Work out the finished part from the listing and answer in its coordinate system (mm). A direction names the side the tool comes from. Coordinates: 2 decimals unless noted, no trailing zeros. Order: outer loops, then holes, each group sorted by start corner. A loop starts at its lowest first (then second) coordinate and runs counter-clockwise, first axis right, second up. Notation, with made-up numbers: M -19,60.5 L 36,60.5 A23 cw 36,90.5 Z; hole C -6,-4 d4. An arc over 180 degrees is marked long. Answer in a Markdown table with one row per item. Add a question column.
Item 1: The mould has two halves that part along Y. Classify faces 1 (the face through (99, 41.6, 10)), 2 (the face through (127.05, 40.93, 8.65)), 3 (the face through (35, 62, 8)): released by +Y, released by -Y, zero draft, split by the parting line, or undercut.
Item 2: The part is cut by section A-A (z = 3.5). Write down the section's boundary in (x, y).
Item 3: Which of the six approach directions +Z, -Z, +X, -X, +Y, -Y give full straight-line access (tool end or side, diameter ignored) to faces 4 (the face through (1.972, 91.669, 8.526)), 5 (the face through (38, 64, 11)), 6 (the face through (125.1, 68.9, 10)), 7 (the face through (9, 102.5, 10))?
Item 4: Flat-ended cylindrical pins translate along their axes: pin 1 Ø3.5 at (y, z) = (99, 13) entering from -X; pin 2 Ø5 at (x, z) = (26, 2) entering from -Y; pin 3 Ø3.5 at (x, y) = (123.5, 98) entering from -Z. Find the tip coordinate at first contact, or state that the pin passes through.
Item 5: Consider line 1 (X direction, y = 87.5, z = 6); line 2 (Y direction, x = 123.4, z = 13.95); line 3 (Y direction, x = 123.4, z = 8). Determine where each line is inside the solid, lowest interval first. Write a range as from..to.
Item 6: The part is cut by section C-C (y = 55.5). Write down the section's boundary in (x, z), then the cut area to 3 significant figures.
Item 7: The part is cut by section D-D (y = 84). Write down the section's boundary in (x, z).
Item 8: The part is cut by section B-B (y = 70.6). Write down the section's boundary in (x, z), then the cut area to 3 significant figures.
from build123d import *

# Parameters (mm, degrees)
SKETCH_R        = 2.25
PAD_DEPTH       = 16
POCKET_DEPTH    = 21
SKETCH002_R     = 1.75
POCKET001_DEPTH = 23
SKETCH003_R     = 1.75
SKETCH003_R_2   = 2.15
POCKET002_DEPTH = 46
SKETCH005_R     = 8
POCKET004_DEPTH = 5
POCKET005_DEPTH = 4.4
SKETCH007_W     = 10.5
SKETCH007_H     = 21
POCKET006_DEPTH = 6
POCKET007_DEPTH = 18
SKETCH009_R     = 1.75
POCKET008_DEPTH = 86


with BuildPart() as part:
    # Sketch → Pad (new body)
    with BuildSketch(Plane.XY):
        with BuildLine():
            Line((126.5, 107.1), (-1.5, 107.1))
            Line((-1.5, 107.1), (-1.5, 104.4))
            Line((-1.5, 104.4), (-5.7, 104.4))
            Line((-5.7, 104.4), (-5.7, 102.4))
            Line((-5.7, 102.4), (0, 102.4))
            Line((0, 102.4), (0, 62))
            Line((0, 62), (70.6, 62))
            Line((70.6, 62), (70.6, 36))
            Line((70.6, 36), (75.6, 36))
            Line((75.6, 36), (133.571068, 36))
            ThreePointArc((133.571068, 36), (133.891989, 37.231735), (134, 38.5))
            Line((134, 38.5), (134, 99.6))
            ThreePointArc((134, 99.6), (131.803301, 104.903301), (126.5, 107.1))
        make_face()
        with Locations((123.4, 70.6)):
            Circle(SKETCH_R, mode=Mode.SUBTRACT)
    extrude(amount=PAD_DEPTH)

    # Sketch001 (on DatumPlane) → Pocket (cut)
    with BuildSketch(Plane.XY.offset(5)):
        Polygon((128.6, 101.8), (131, 101.8), (131, 79.9), (120.7, 79.9), (120.7, 93.6), (120.7, 93.9), (124.3, 93.9), (128.6, 93.9), align=None)
        with BuildLine():
            add(Edge.make_bspline(
                [(13.289069, 102.5), (27.487875, 102.5), (63.575842, 75.600151), (81.110251, 102.5), (98.331885, 102.5)],
                knots=[0, 0, 0, 0, 0.5, 1, 1, 1, 1], degree=3))
            Line((98.331885, 102.5), (109.7, 102.5))
            Line((109.7, 102.5), (109.7, 58))
            Line((109.7, 58), (122, 58))
            Line((122, 58), (122, 41.6))
            Line((122, 41.6), (80, 41.6))
            Line((80, 41.6), (75.6, 41.6))
            Line((75.6, 41.6), (75.6, 67))
            Line((75.6, 67), (4, 67))
            Line((4, 67), (4, 102.5))
            Line((4, 102.5), (13.289069, 102.5))
        make_face()
    extrude(amount=POCKET_DEPTH, mode=Mode.SUBTRACT)

    # Sketch002 → Pocket001 (cut)
    with BuildSketch(Plane.YZ):
        with Locations((12, 8)):
            Circle(SKETCH002_R)
        with Locations((60, 8)):
            Circle(SKETCH002_R)
        with Locations((90, 8)):
            Circle(SKETCH002_R)
    extrude(amount=POCKET001_DEPTH, mode=Mode.SUBTRACT)

    # Sketch003 → Pocket002 (cut)
    with BuildSketch(Plane.XZ):
        with Locations((58.6, 8)):
            Circle(SKETCH003_R)
        with Locations((8, 8)):
            Circle(SKETCH003_R)
        with Locations((125, 8)):
            Circle(SKETCH003_R_2)
    extrude(amount=-POCKET002_DEPTH, mode=Mode.SUBTRACT)

    # Sketch005 (on DatumPlane) → Pocket004 (cut, symmetric)
    with BuildSketch(Plane.XY.offset(5)):
        with Locations((123.4, 70.6)):
            Circle(SKETCH005_R)
    extrude(amount=POCKET004_DEPTH, both=True, mode=Mode.SUBTRACT)

    # Sketch006 (on DatumPlane) → Pocket005 (cut)
    with BuildSketch(Plane.XY.offset(16)):
        Polygon((116.7, 102.3), (124.3, 102.3), (124.3, 93.9), (124.3, 93.6), (120.7, 93.6), (116.7, 93.6), align=None)
    extrude(amount=-POCKET005_DEPTH, mode=Mode.SUBTRACT)

    # Sketch007 (on DatumPlane) → Pocket006 (cut)
    with BuildSketch(Plane.XY.offset(5)):
        with Locations((125.75, 91.3)):
            Rectangle(SKETCH007_W, SKETCH007_H)
    extrude(amount=-POCKET006_DEPTH, mode=Mode.SUBTRACT)

    # Sketch008 (on DatumPlane) → Pocket007 (cut)
    with BuildSketch(Plane.XY.offset(5)):
        Polygon((127.328613, 102.8), (132, 102.8), (132, 79.494476), (119.5, 79.494476), (119.5, 94.960373), (127.328613, 94.960373), align=None)
    extrude(amount=POCKET007_DEPTH, mode=Mode.SUBTRACT)

    # Sketch009 → Pocket008 (cut)
    with BuildSketch(Plane.XZ):
        with Locations((58.6, 8)):
            Circle(SKETCH009_R)
        with BuildLine():
            ThreePointArc((33, 16), (38, 11), (43, 16))
            Line((43, 16), (43, 31.673506))
            ThreePointArc((43, 31.673506), (38, 36.673506), (33, 31.673506))
            Line((33, 31.673506), (33, 16))
        make_face()
    extrude(amount=-POCKET008_DEPTH, mode=Mode.SUBTRACT)


solid = part.part
Reply:
| question | item | result |
|---|---|---|
| 1 | face 1 | undercut |
| 1 | face 2 | zero draft |
| 1 | face 3 | released by -Y |
| 2 | outline | M -5.7,102.4 L 0,102.4 L 0,62 L 70.6,62 L 70.6,36 L 133.57,36 A7.5 ccw 134,38.5 L 134,99.6 A7.5 ccw 126.5,107.1 L -1.5,107.1 L -1.5,104.4 L -5.7,104.4 Z; hole C 123.4,70.6 d16; hole M 120.5,80.8 L 131,80.8 L 131,101.8 L 120.5,101.8 Z |
| 3 | face 4 | -X |
| 3 | face 5 | +Z, -Y |
| 3 | face 6 | -Z |
| 3 | face 7 | +Z |
| 4 | pin 1 | stops at x = 0 |
| 4 | pin 2 | stops at y = 62 |
| 4 | pin 3 | stops at z = 5 |
| 5 | line 1 | x = 0..4, 109.7..119.5, 132..134 |
| 5 | line 2 | y = 36..68.35, 72.85..79.49, 102.3..107.1 |
| 5 | line 3 | y = 46..62.6, 78.6..79.49, 94.96..107.1 |
| 6 | outline | M 70.6,0 L 134,0 L 134,16 L 122,16 L 122,5 L 75.6,5 L 75.6,16 L 70.6,16 Z |
| 6 | area | 504 mm2 |
| 7 | outline | M 0,0 L 120.5,0 L 120.5,5 L 119.5,5 L 119.5,16 L 109.7,16 L 109.7,5 L 4,5 L 4,16 L 0,16 Z; M 131,0 L 134,0 L 134,16 L 132,16 L 132,5 L 131,5 Z |
| 8 | outline | M 0,0 L 115.4,0 L 115.4,10 L 121.15,10 L 121.15,16 L 109.7,16 L 109.7,5 L 4,5 L 4,16 L 0,16 Z; M 125.65,10 L 131.4,10 L 131.4,0 L 134,0 L 134,16 L 125.65,16 Z |
| 8 | area | 794 mm2 |
